The figure shows three views and two pictorial views of one solid part (mm, origin at its lowest corner). Answer the questions. A direction names the side the tool comes from. Coordinates: 2 decimals unless noted, no trailing zeros. Order: outer loops, then holes, each group sorted by start corner. A loop starts at its lowest first (then second) coordinate and runs counter-clockwise, first axis right, second up. Notation, with made-up numbers: (89.5, 22.25) -> (128.5, 22.25) arc R20 ccw to (128.5, 39.25) -> close; hole circle Ø9 at (20.25, 40). An arc over 180 degrees is marked (long way). Return JSON: item names as keys, results as strings.
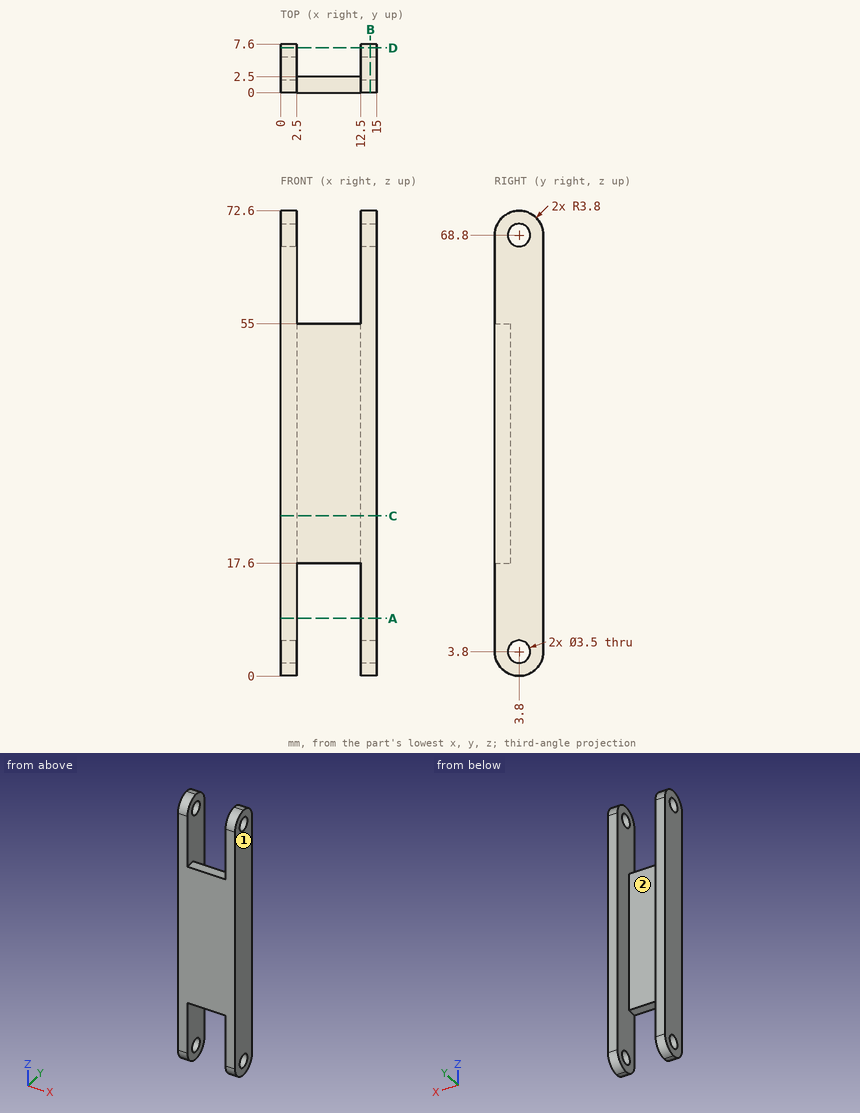
1. The part is cut by section A-A on z = 9. Give the vertices of the cut face in (x, y), and give its area (3 significant figures).
Answer block:
{"outline": "(0, 0) -> (2.5, 0) -> (2.5, 7.6) -> (0, 7.6) -> close; (12.5, 0) -> (15, 0) -> (15, 7.6) -> (12.5, 7.6) -> close", "area": "38.0 mm2"}
2. The part is cut by section D-D on y = 7. Give the vertices of the cut face in (x, z), and give its area (3 significant figures).
Answer block:
{"outline": "(0, 1.75) -> (2.5, 1.75) -> (2.5, 70.85) -> (0, 70.85) -> close; (12.5, 1.75) -> (15, 1.75) -> (15, 70.85) -> (12.5, 70.85) -> close", "area": "345 mm2"}
3. Consider line 1 (X direction, y = 2.5, z = 7.5); line 2 (Z direction, x = 1.25, y = 4.25); line 3 (Y direction, x = 10, z = 49). Determine where each line is inside the solid, lowest interval first. Write a range as from..to.
Answer block:
{"line 1": "x = 0..2.5, 12.5..15", "line 2": "z = 0.03..2.11, 5.49..67.11, 70.49..72.57", "line 3": "y = 0..2.5"}
4. The part is cut by section C-C on z = 25. Give the vertices of the cut face in (x, y).
Answer block:
{"outline": "(0, 0) -> (15, 0) -> (15, 7.6) -> (12.5, 7.6) -> (12.5, 2.5) -> (2.5, 2.5) -> (2.5, 7.6) -> (0, 7.6) -> close"}
5. Each of these flat-tipped pins is pushed along its axis until it touches: pin 1 Ø3 at (x, z) = (6, 19) entering from +Y; pin 2 Ø3 at (x, y) = (5, 1) entering from +Z; pin 3 Ø2 at (x, y) = (9, 1) entering from -Z. Where does it stop, or does it pass through?
Answer block:
{"pin 1": "stops at y = 2.5", "pin 2": "stops at z = 55", "pin 3": "stops at z = 17.6"}
6. For the marked faces 1 and 2, determine the directions among +Z, -Z, +X, -X, +Y, -Y from which every point of the face is accessible in a straight line to the end or side of a thin tool.
Answer block:
{"face 1": "+Z, -Z, +X, +Y, -Y", "face 2": "+Z, -Z, +Y"}
7. The part is cut by section B-B on x = 14. Give the vertices of the cut face in (y, z), and give its area (3 significant figures).
Answer block:
{"outline": "(0, 3.8) arc R3.8 ccw to (3.8, 0) arc R3.8 ccw to (7.6, 3.8) -> (7.6, 68.8) arc R3.8 ccw to (3.8, 72.6) arc R3.8 ccw to (0, 68.8) -> close; hole circle Ø3.5 at (3.8, 3.8); hole circle Ø3.5 at (3.8, 68.8)", "area": "520 mm2"}
